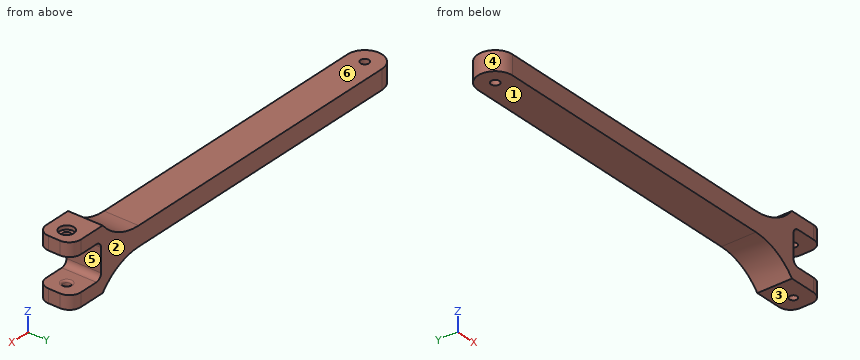
from build123d import *

# Parameters (mm, degrees)
SKETCH1_R           = 1.1
BOSS_EXTRUDE1_DEPTH = 5
BOSS_EXTRUDE2_DEPTH = 9
FILLET1_R           = 15
SKETCH3_R           = 1
CUT_EXTRUDE1_DEPTH  = 16
FILLET2_R           = 3
SKETCH4_R           = 1.9
CUT_EXTRUDE2_DEPTH  = 1
FILLET3_R           = 1.5
FILLET4_R           = 0.5


with BuildPart() as part:
    # Sketch1 → Boss-Extrude1 (new body)
    with BuildSketch(Plane.XY):
        with BuildLine():
            ThreePointArc((0, 4.5), (-4.5, 0), (0, -4.5))
            Line((0, -4.5), (90, -4.5))
            Line((90, -4.5), (90, 4.5))
            Line((90, 4.5), (0, 4.5))
        make_face()
        Circle(SKETCH1_R, mode=Mode.SUBTRACT)
    extrude(amount=BOSS_EXTRUDE1_DEPTH)

    # Sketch2 → Boss-Extrude2 (add)
    with BuildSketch(Plane(origin=(0, 4.5, 0), x_dir=(1, 0, 0), z_dir=(0, 1, 0))):
        Polygon((90.5, 2), (100, 2), (100, 5.5), (90, 5.5), (90, 0), (90, -5), (90, -10.5), (100, -10.5), (100, -7), (90.5, -7), align=None)
    extrude(amount=-BOSS_EXTRUDE2_DEPTH)

    # Fillet1
    # the kernel refuses this fillet: 15 mm, written as the material it adds along each edge
    with BuildSketch(Plane(origin=(90, -4.5, 0), x_dir=(0, 0, -1), z_dir=(0, 1, 0))) as fillet1_piece_1:
        with BuildLine():
            CenterArc((15, 11.608186766), FILLET1_R, 180, 50.703519761)
            Line((0, 11.608186766), (-0.3, 11.608186766))
            Line((-0.3, 11.608186766), (-0.3, 0))
            Line((-0.3, 0), (0, -0.3))
            ThreePointArc((0, -0.3), (2.75, -0.3), (5.31, -0.232163735))
            Line((5.31, -0.232163735), (5.5, 0))
        make_face()
    extrude(amount=9)
    with BuildSketch(Plane(origin=(90, -4.5, 5), x_dir=(0, 0, 1), z_dir=(0, 1, 0))) as fillet1_piece_2:
        with BuildLine():
            CenterArc((15, -11.608186766), FILLET1_R, 129.296480239, 50.703519761)
            Line((0, -11.608186766), (-0.3, -11.608186766))
            Line((-0.3, -11.608186766), (-0.3, 0))
            Line((-0.3, 0), (0, 0.3))
            ThreePointArc((0, 0.3), (2.75, 0.3), (5.31, 0.232163735))
            Line((5.31, 0.232163735), (5.5, 0))
        make_face()
    extrude(amount=9)

    # Sketch3 → Cut-Extrude1 (cut)
    with BuildSketch(Plane.XY.offset(10.5)):
        with Locations((96, 0)):
            Circle(SKETCH3_R)
    extrude(amount=-CUT_EXTRUDE1_DEPTH, mode=Mode.SUBTRACT)

    # Fillet2
    fillet2_edges = [part.edges().sort_by_distance(p)[0] for p in [
        (100, 4.5, 8.75),
        (100, 4.5, -3.75),
        (100, -4.5, 8.75),
        (100, -4.5, -3.75),
    ]]
    fillet(fillet2_edges, radius=FILLET2_R)

    # Sketch4 → Cut-Extrude2 (cut)
    with BuildSketch(Plane.XY.offset(10.5)):
        with Locations((96, 0)):
            Circle(SKETCH4_R)
    extrude(amount=-CUT_EXTRUDE2_DEPTH, mode=Mode.SUBTRACT)

    # Fillet3
    fillet3_edges = [part.edges().sort_by_distance(p)[0] for p in [
        (90.5, 0, 7),
        (90.5, 0, -2),
    ]]
    fillet(fillet3_edges, radius=FILLET3_R)

    # Fillet4
    fillet4_edges = [part.edges().sort_by_distance(p)[0] for p in [
        (95, 0, -2),
    ]]
    fillet(fillet4_edges, radius=FILLET4_R)


solid = part.part
Can you work these out from the model? Positions are in its coordinate system, mm. Face numbers are marked on the shaded views. A direction names the side the tool comes from. Coordinates: 2 decimals unless noted, no trailing zeros. Write each loop counter-clockwise with the first axis right and the second up, starting at its lowest first coordinate (ties: lowest second). Pieces come first, ordered by that corner, then holes. Notation, with made-up numbers: (-28, -19) - (-1, -19) arc R29 ccw to (-1, 10) - close; hole circle Ø3 at (-12.75, 82). An arc over 180 degrees is marked (long way). Return JSON: item names as keys, results as strings. Group by question number.
Item 1: If we section it at D-D (x = 32.5): Write out the boundary of the cut face in (y, z), then the cut area to 3 significant figures.
Item 2: Please list where these lines run through material, in increasing order: probe 1 along Y at (x, z) = (96, -3.9); probe 2 along Z at (x, y) = (14, 3); probe 3 along X at (y, z) = (0.75, -3).
Item 3: We'd pull the mould along Z, two halves only. Please class the marked faces 3, 4, 5 and 6: pulls with the +Z half, pulls with the -Z half, needs draft (parallel to the pull), parting line crosses it, or undercut.
Item 4: Which directions (+Z, -Z, +X, -X, +Y, -Y) give clear straight access to the entire face, cutting with the end or side of a thin tool? Please do the marked faces 1 and 2.
Item 5: If we section it at C-C (z = 3): Write out the boundary of the cut face in (x, y), then the cut area to 3 significant figures.
Item 6: If we section it at A-A (y = 0): Count the separate pieces of the cut face and the enclosed holes in it, then the cut area to 3 significant figures.
Item 7: I'm going to push flat-ended pins straight in: pin 1 Ø2.5 at (x, y) = (27.5, -2) entering from -Z; pin 2 Ø1.6 at (x, y) = (96, 0) entering from +Z; pin 3 Ø5 at (y, z) = (0, 2.5) entering from +X; pin 4 Ø1.9 at (x, y) = (96.5, 0.5) entering from +Z. Where does each tip first touch, or does it pass through?
Item 8: If we section it at B-B (x = 96): Write out the boundary of the cut face in (y, z).
Return value:
{
 "1": {"outline": "(-4.5, 0) - (4.5, 0) - (4.5, 5) - (-4.5, 5) - close", "area": "45.0 mm^2"},
 "2": {"probe 1": "y = -4.5 to -1, 1 to 4.5", "probe 2": "z = 0 to 5", "probe 3": "x = 87.39 to 95.34, 96.66 to 100"},
 "3": {"face 3": "pulls with the -Z half", "face 4": "needs draft", "face 5": "undercut", "face 6": "pulls with the +Z half"},
 "4": {"face 1": "-Z, -X, +Y, -Y", "face 2": "+Z, -Z, +X, -X, +Y"},
 "5": {"outline": "(0, -4.5) - (90.5, -4.5) - (90.5, 4.5) - (0, 4.5) arc R4.5 ccw to start; hole circle Ø2.2 at (0, 0)", "area": "843 mm^2"},
 "6": {"separate pieces": "4", "enclosed holes": "0", "area": "560 mm^2"},
 "7": {"pin 1": "stops at z = 0", "pin 2": "passes through", "pin 3": "stops at x = 90.5", "pin 4": "stops at z = 9.5"},
 "8": {"outline": "(-4.5, -5.5) - (-1, -5.5) - (-1, -2.5) arc R0.5 ccw to (-1.5, -2) - (-4.5, -2) - close; (-4.5, 7) - (-1, 7) - (-1, 9.5) - (-1.9, 9.5) - (-1.9, 10.5) - (-4.5, 10.5) - close; (1, -5.5) - (4.5, -5.5) - (4.5, -2) - (1.5, -2) arc R0.5 ccw to (1, -2.5) - close; (1, 7) - (4.5, 7) - (4.5, 10.5) - (1.9, 10.5) - (1.9, 9.5) - (1, 9.5) - close"}
}
